Autodesk Fusion 360 part; units mm, degrees
sketch "BaseA3" plane through (0, 0, 0) normal (0, 0, 1) x (1, 0, 0)
  line L0 (0, 0) -> (28, 0)
  line L1 (28, 88) -> (0, 88)
  line L2 (0, 0) -> (-3, 0)
  line L3 (-3, 88) -> (0, 88)
  line L4 (-3, 0) -> (-16, 0)
  line L5 (-16, 88) -> (-3, 88)
  line L6 (-9.5, 0) -> (-9.5, 44) construction
  line L7 (-9.5, 44) -> (-16, 44) construction
  line L8 (-16, 44) -> (-22, 44) construction
  circle A0 centre (-22, 44) radius 9.5
  arc A1 (-22, 63) -> (-22, 25) centre (-22, 44) ccw
  line L9 (-16, 0) -> (-16, 19)
  line L10 (-16, 69) -> (-16, 88)
  arc A2 (-22, 63) -> (-16, 69) centre (-22, 69) ccw
  arc A3 (-16, 19) -> (-22, 25) centre (-22, 19) ccw
  line L11 (0, 63) -> (0, 63)
  line L12 (0, 25) -> (0, 22) construction
  line L13 (0, 22) -> (-3, 22) construction
  arc A4 (0, 25) -> (-3, 22) centre (0, 22) ccw
  line L14 (-9.5, 44) -> (0, 44) construction
  arc A5 (-3, 66) -> (0, 63) centre (0, 66) ccw
  line L15 (-22, 69) -> (-22, 63) construction
  line L16 (-22, 69) -> (-16, 69) construction
  line L17 (-22, 63) -> (-22, 25) construction
  line L18 (-22, 25) -> (-22, 19) construction
  line L19 (-22, 19) -> (-16, 19) construction
  line L20 (0, 63) -> (0, 66) construction
  line L21 (0, 66) -> (-3, 66) construction
  line L22 (-3, 69) -> (28, 69) construction
  circle A6 centre (28, 69) radius 5
  line L23 (0, 44) -> (28, 44) construction
  circle A7 centre (28, 19) radius 5
  line L24 (-3, 19) -> (28, 19) construction
  line L25 (28, 19) -> (64, 19) construction
  line L26 (64, 19) -> (64, 69) construction
  line L27 (64, 69) -> (28, 69) construction
  line L28 (28, 0) -> (46.834, 0)
  line L29 (46.834, 0) -> (64, 17.146)
  line L30 (64, 17.146) -> (77.427, 30.5569)
  line L31 (28, 44) -> (83, 44) construction
  line L32 (64, 70.854) -> (77.427, 57.4431)
  line L33 (46.834, 88) -> (64, 70.854)
  line L34 (28, 88) -> (46.834, 88)
  arc A8 (77.427, 30.5569) -> (77.427, 57.4431) centre (64, 44) ccw
  line L35 (-3, 88) -> (-3, 66)
  line L36 (-3, 22) -> (-3, 0)
  line L37 (-3, 0) -> (-3, 22)
  line L38 (-3, 66) -> (-3, 88)
  line L39 (0, 49) -> (1, 49)
  line L40 (1, 49) -> (1, 39)
  line L41 (1, 39) -> (0, 39)
  line L42 (0, 63) -> (0, 49)
  line L43 (0, 39) -> (0, 25)
  dimension "d3" = 13
  dimension "d4" = 88
  dimension "d5" = 19
extrude "Extrude1" add sketch "BaseA3" along normal blind 10 contours L0 L1 L2 L3 A4 A5 L28 L29 L30 L32 L33 L34 A8 L35 L36 L37 L38 L39 L40 L41 L42 L43
extrude "Extrude2" add sketch "BaseA3" along normal blind 50 contours L4 L5 A1 L9 L10 A2 A3 A4 A5 L35 L36 L37 L38 L39 L40 L41 L42 L43
fillet "Fillet1" radius 13 1 edges at (46.834, 0, 5)
fillet "Fillet2" radius 13 1 edges at (46.834, 88, 5)
sketch "Triangle" plane through (0, 0, 0) normal (0, -1, 0) x (1, 0, 0)
  line L0 (41.4537, 0) -> (41.4537, 10)
  line L1 (41.4537, 10) -> (-3, 10)
  line L2 (-3, 10) -> (-3, 50)
  line L3 (-3, 50) -> (-16, 50)
  line L4 (-16, 50) -> (-16, 0)
  line L5 (-16, 0) -> (41.4537, 0)
  line L6 (-3, 10) -> (1, 10)
  line L7 (1, 50) -> (1, 10)
  line L8 (1, 10) -> (68, 10)
  line L9 (68, 10) -> (1, 50)
extrude "Extrude3" add sketch "Triangle" against normal blind 10 from surface at -39 contours L1 L7 L8 L9
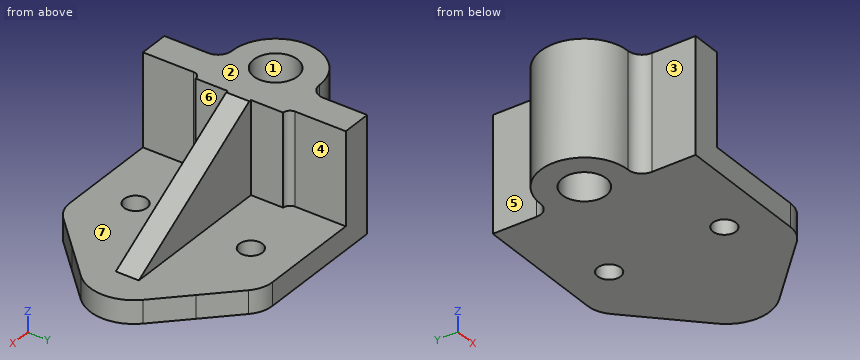
The model under review builds one solid part; all positions refer to its coordinate system, in mm. Face numbers are marked on the shaded views. A direction names the side the tool comes from. Round coordinates to 2 decimals unless told otherwise and drop trailing zeros. Loops run counter-clockwise (first coordinate to the right, second up) from the corner with the lowest first, then second, coordinate; pieces in that order, holes last. Notation, with made-up numbers: M 53,42.5 L 58,42.5 A23 ccw 58,81.5 Z; hole C 10.5,64 d8. An arc over 180 degrees is marked long. Answer as CSV lines item,"result". Start each with the question number.
Item 1: Consider section B-B (x = -14). Write out the cut boundary in (y, z), then the cut area to 3 significant figures.
Item 2: Wall thickness on line 1 (Y direction, x = 28, z = 5); line 2 (Y direction, x = -22, z = 27); line 3 (Y direction, x = 17, z = 37): over which ranges is each line inside the solid? List them lowest first. Write a range as [from, to].
Item 3: Consider section A-A (z = 22). Write out the cut boundary in (x, y).
Item 4: Mouldability with a two-part tool opening along X and no side actions: class the marked faces 1, 2 and 3 as released by +X, released by -X, zero draft, split by the parting line, or undercut.
Item 5: For the marked faces 4, 5, 6 and 7, list the 3-axis set-ups (+Z, -Z, +X, -X, +Y, -Y) from which the entire face can be reached by the end or side of a thin tool; tool diameter is ignored.
Item 6: Consider section C-C (y = 37.5). Write out the cut boundary in (x, z), then the cut area to 3 significant figures.
Item 7: Consider section D-D (x = 28). Write out the cut boundary in (y, z), then the cut area to 3 significant figures.
Item 8: Insertion check: P1, Ø1.5, axis at y = 62, z = 23.5, coming from the -X side; P2, Ø10, axis at x = 69, y = 59.5, coming from the +Z side; P3, Ø4, axis at y = 59, z = 32, coming from the +X side. Each pin has a flat end and moves straight along its axis. Give the tip position at first contact, or say it passes through.
Answer:
1,outline,"M 0,0 L 38.88,0 L 38.88,50 L 0,50 Z; M 49.12,0 L 88,0 L 88,50 L 49.12,50 Z"
1,area,"3,890 mm^2"
2,line 1,"y = [0, 14], [24, 64], [74, 88]"
2,line 2,"y = [25, 34.5], [53.5, 63]"
2,line 3,"y = [39, 49]"
3,outline,"M -22,25 A6 cw -16,19 L -16,0 L -3,0 L -3,22 A3 cw 0,25 L 0,39 L 47.9,39 L 47.9,49 L 0,49 L 0,63 A3 cw -3,66 L -3,88 L -16,88 L -16,69 A6 cw -22,63 A19 ccw Z; hole C -22,44 d19"
4,face 1,"undercut"
4,face 2,"zero draft"
4,face 3,"released by -X"
5,face 4,"+Z, +X, +Y"
5,face 5,"+Z, -Z, -X, +Y"
5,face 6,"+Z, +X, -Y"
5,face 7,"+Z, +X"
6,outline,"M -39.85,0 L -28.93,0 L -28.93,50 L -39.85,50 Z; M -15.07,0 L 81.85,0 L 81.85,10 L 0,10 L 0,50 L -15.07,50 Z"
6,area,"2,120 mm^2"
7,outline,"M 0,0 L 14,0 L 14,10 L 0,10 Z; M 24,0 L 64,0 L 64,10 L 49,10 L 49,33.88 L 39,33.88 L 39,10 L 24,10 Z; M 74,0 L 88,0 L 88,10 L 74,10 Z"
7,area,"919 mm^2"
8,P1,"stops at x = -29.96"
8,P2,"stops at z = 10"
8,P3,"stops at x = 0"
